from build123d import *

# Parameters (mm, degrees)
SKETCH1_R           = 37.5
BOSS_EXTRUDE1_DEPTH = 579.5
SKETCH2_R           = 75
BOSS_EXTRUDE2_DEPTH = 200
SKETCH3_R           = 25
CUT_EXTRUDE1_DEPTH  = 100
SKETCH4_W           = 260.945871841
SKETCH4_H           = 75.746474917
CUT_EXTRUDE2_DEPTH  = 100


with BuildPart() as part:
    # Sketch1 → Boss-Extrude1 (new, symmetric)
    with BuildSketch(Plane.XY):
        Circle(SKETCH1_R)
    extrude(amount=BOSS_EXTRUDE1_DEPTH, both=True)

    # Sketch2 → Boss-Extrude2 (add)
    with BuildSketch(Plane(origin=(0, 0, -579.5), x_dir=(-1, 0, 0), z_dir=(0, 0, -1))):
        Circle(SKETCH2_R)
    extrude(amount=BOSS_EXTRUDE2_DEPTH)

    # Sketch3 → Cut-Extrude1 (cut, symmetric)
    with BuildSketch(Plane(origin=(0, 0, 0), x_dir=(1, 0, 0), z_dir=(0, 1, 0))):
        with Locations(Location((0, 719.26, 0), (0, 0, 270))):
            Circle(SKETCH3_R)
        with BuildLine():
            Line((60.24, 719.26), (60.24, 646.55))
            Line((60.24, 646.55), (75, 579.5))
            Line((75, 579.5), (150.12522471, 579.5))
            Line((150.12522471, 579.5), (155.105572786, 831.544185687))
            Line((155.105572786, 831.544185687), (-155.801518438, 837.687654259))
            Line((-155.801518438, 837.687654259), (-75, 579.5))
            Line((-75, 579.5), (-60.24, 646.55))
            Line((-60.24, 646.55), (-60.24, 719.26))
            ThreePointArc((-60.24, 719.26), (0, 779.5), (60.24, 719.26))
        make_face()
    extrude(amount=CUT_EXTRUDE1_DEPTH, both=True, mode=Mode.SUBTRACT)

    # Sketch4 → Cut-Extrude2 (cut, symmetric)
    with BuildSketch(Plane(origin=(60.24, 0, 0), x_dir=(0, 0, -1), z_dir=(1, 0, 0))):
        with Locations((730.83293592, 100.543237459)):
            Rectangle(SKETCH4_W, SKETCH4_H)
        with Locations((730.83293592, -100.543237459)):
            Rectangle(SKETCH4_W, SKETCH4_H)
    extrude(amount=CUT_EXTRUDE2_DEPTH, both=True, mode=Mode.SUBTRACT)


solid = part.part
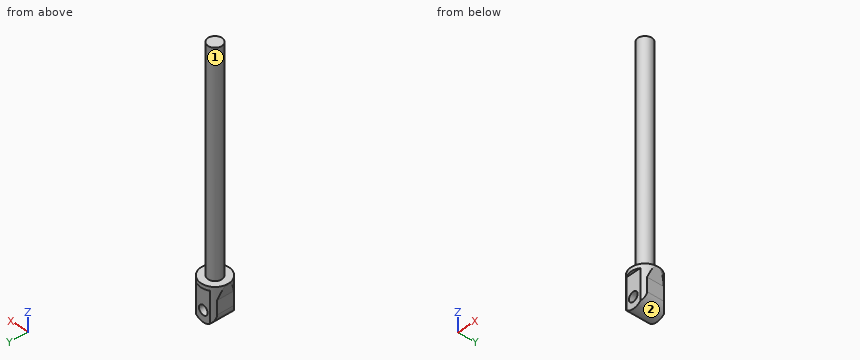
Verification items for the finished model (mm, model axes). Face numbers are marked on the shaded views. A direction names the side the tool comes from. Coordinates: 2 decimals unless noted, no trailing zeros. Loops run counter-clockwise (first coordinate to the right, second up) from the corner with the lowest first, then second, coordinate; pieces in that order, holes last. Notation, with made-up numbers: M 35,-8 L 68,-8 A15 ccw 68,4 Z; hole C 55,64 d11. An arc over 180 degrees is marked long. One line per item, written item: value.
1. Section check A-A on x = 0. Record the cut outline in (y, z).
Answers follow:
outline: M -75,-600.36 L -62.67,-600.36 L -62.67,-694.26 L 62.67,-694.26 L 62.67,-600.36 L 75,-600.36 L 75,-579.5 L 37.5,-579.5 L 37.5,579.5 L -37.5,579.5 L -37.5,-579.5 L -75,-579.5 Z; M -62.67,-779.5 L 62.67,-779.5 L 62.67,-744.26 L -62.67,-744.26 Z
2. Set-up check for the marked faces 1 and 2: record each of +Z, -Z, +X, -X, +Y, -Y from which the full face is reachable in a straight line by a thin tool's end or side.
Answers follow:
face 1: +Z
face 2: -Z, +Y, -Y
3. Gauge pin test, flat ends, axial feed: P1, Ø6, axis at y = -35, z = -55, coming from the +X side; P2, Ø13.5, axis at x = 12, y = 66.5, coming from the -Z side; P3, Ø0.5, axis at y = -63.5, z = -642, coming from the +X side. Record the tip position at first contact, or that the pin passes through.
Answers follow:
P1: x = 19.55
P2: z = -779.15
P3: x = -39.76
4. Section check B-B on z = -304.5. Record the cut outline in (x, y), plus the area to 3 significant figures.
Answers follow:
outline: C 0,0 d75
area: 4,420 mm^2
5. Material ranges on line 1 along Z through (x, y) = (0, 39); line 2 along X through (y, z) = (32, -719); line 3 along Z through (x, y) = (0, 16.5), recorded low to high. Write a range as from..to.
Answers follow:
line 1: -779.5..-744.26, -694.26..-579.5
line 2: -60.24..-25, 25..60.24
line 3: -779.5..-744.26, -694.26..579.5
